Work out the finished part from the listing and answer in its coordinate system (mm). Coordinates: 2 decimals unless noted, no trailing zeros. Loops run counter-clockwise (first coordinate to the right, second up) from the corner with the lowest first, then second, coordinate; pieces in that order, holes last. Notation, with made-up numbers: (20, -6.5) -> (24, -6.5) arc R28 ccw to (24, 11.5) -> close; hole circle Ø1 at (37.25, 81). An arc over 180 degrees is marked (long way). Answer as CSV lines item,"result".
```python
from build123d import *

# Parameters (mm, degrees)
SKETCH_W     = 88.9
SKETCH_H     = 50.8
SKETCH_R     = 2.5
SKETCH_W_2   = 9
SKETCH_H_2   = 9
PAD_DEPTH    = 4
SKETCH001_R  = 6
PAD001_DEPTH = 88.9
FILLET_R     = 4
CHAMFER_SIZE = 1.5


with BuildPart() as part:
    # Sketch → Pad (new body)
    with BuildSketch(Plane.XY):
        with Locations((44.45, 25.4)):
            Rectangle(SKETCH_W, SKETCH_H)
        with Locations((15.45, 8)):
            Circle(SKETCH_R, mode=Mode.SUBTRACT)
        with Locations((73.45, 8)):
            Circle(SKETCH_R, mode=Mode.SUBTRACT)
        with Locations((6.45, 30)):
            Circle(SKETCH_R, mode=Mode.SUBTRACT)
        with Locations((82.45, 30)):
            Circle(SKETCH_R, mode=Mode.SUBTRACT)
        with Locations((44.45, 14.5)):
            Rectangle(SKETCH_W_2, SKETCH_H_2, mode=Mode.SUBTRACT)
    extrude(amount=PAD_DEPTH)

    # Sketch001 (on Face4 of Pad) → Pad001 (join)
    with BuildSketch(Plane(origin=(0, 0, 0), x_dir=(0, -1, 0), z_dir=(-1, 0, 0))):
        with BuildLine():
            Line((-50.8, 0), (-56.8, 0))
            Line((-56.8, 0), (-59.623533, 5.294124))
            ThreePointArc((-50.8, 0), (-45.655039, 18.574927), (-59.623533, 5.294124))
        make_face()
        with Locations((-50.8, 10)):
            Circle(SKETCH001_R, mode=Mode.SUBTRACT)
    extrude(amount=-PAD001_DEPTH)

    # Fillet
    fillet_edges = [part.edges().sort_by_distance(p)[0] for p in [
        (44.45, 42.8, 4),
    ]]
    fillet(fillet_edges, radius=FILLET_R)

    # Chamfer
    chamfer_edges = [part.edges().sort_by_distance(p)[0] for p in [
        (79.95, 30, 4),
        (3.95, 30, 4),
        (70.95, 8, 0),
        (12.95, 8, 0),
        (44.45, 10, 0),
        (39.95, 14.5, 0),
        (44.45, 19, 0),
        (48.95, 14.5, 0),
        (39.95, 14.5, 4),
        (44.45, 19, 4),
        (48.95, 14.5, 4),
        (44.45, 10, 4),
    ]]
    chamfer(chamfer_edges, length=CHAMFER_SIZE)


solid = part.part
```
(1) For a pull along Z with two mould halves and no side action, classify faces 1 (the face through (44, 28, 0)), 2 (the face through (43.83, 45.26, 7.7)), 3 (the face through (44, 23, 4)), 4 (the face through (14.91, 5.56, 2.73)) as pulls with the +Z half, pulls with the -Z half, needs draft (parallel to the pull), parting line crosses it, or undercut.
Computed values:
face 1,"pulls with the -Z half"
face 2,"undercut"
face 3,"pulls with the +Z half"
face 4,"needs draft"
(2) A cutting plane is placed at B-B, the plane x = 6.45. Write down the section's boundary in (y, z), and give its area (3 significant figures).
Computed values:
outline,"(0, 0) -> (27.5, 0) -> (27.5, 2.5) -> (26, 4) -> (0, 4) -> close; (32.5, 0) -> (56.8, 0) -> (59.62, 5.29) arc R10 ccw (long way) to (40.9, 8.57) arc R4 cw to (36.94, 4) -> (34, 4) -> (32.5, 2.5) -> close; hole circle Ø12 at (50.8, 10)"
area,"372 mm2"
(3) Consider line 1 along Y through (x, z) = (49.5, 10); line 2 along Z through (x, y) = (26, 50.8); line 3 along Z through (x, y) = (70.5, 20.5). Determine where each line is inside the solid, lowest interval first.
Computed values:
line 1,"40.8 to 44.8, 56.8 to 60.8"
line 2,"0 to 4, 16 to 20"
line 3,"0 to 4"
(4) A cutting plane is placed at D-D, the plane x = 63. Write down the section's boundary in (y, z), and give its area (3 significant figures).
Computed values:
outline,"(0, 0) -> (56.8, 0) -> (59.62, 5.29) arc R10 ccw (long way) to (40.9, 8.57) arc R4 cw to (36.94, 4) -> (0, 4) -> close; hole circle Ø12 at (50.8, 10)"
area,"394 mm2"
(5) A cutting plane is placed at A-A, the plane z = 10. Write down the section's boundary in (x, y), and give its area (3 significant figures).
Computed values:
outline,"(0, 40.8) -> (88.9, 40.8) -> (88.9, 44.8) -> (0, 44.8) -> close; (0, 56.8) -> (88.9, 56.8) -> (88.9, 60.8) -> (0, 60.8) -> close"
area,"711 mm2"
(6) Flat-ended cylindrical pins translate along their axes: pin 1 Ø5 at (x, z) = (30.5, 12) entering from +Y; pin 2 Ø6.5 at (x, y) = (82.45, 30) entering from +Z; pin 3 Ø12 at (x, y) = (52.5, 7.5) entering from +Z; pin 4 Ø3 at (x, z) = (56.5, 17.5) entering from -Y. Find the tip coordinate at first contact, or state that the pin passes through.
Computed values:
pin 1,"y = 60.8"
pin 2,"z = 3.25"
pin 3,"z = 4"
pin 4,"y = 42.8"
(7) A cutting plane is placed at C-C, the plane y = 50.8. Write down the section's boundary in (x, z).
Computed values:
outline,"(0, 0) -> (88.9, 0) -> (88.9, 4) -> (0, 4) -> close; (0, 16) -> (88.9, 16) -> (88.9, 20) -> (0, 20) -> close"
